For this review, take the finished solid that the model builds, in its own axes (mm). A direction names the side the tool comes from. Coordinates: 2 decimals unless noted, no trailing zeros. Order: outer loops, then holes, each group sorted by start corner. A loop starts at its lowest first (then second) coordinate and runs counter-clockwise, first axis right, second up. Notation, with made-up numbers: (34.25, -29) -> (88.25, -29) arc R27 cw to (88.25, -12) -> close; hole circle Ø5 at (-6, 84.25). An arc over 180 degrees is marked (long way). Return JSON: item names as keys, results as strings. Group by question number.
Item 1: Take a section at A-A (y = -5). Write out the cut boundary in (x, z).
Item 2: Take a section at D-D (z = 16.5). Write out the cut boundary in (x, y), then the cut area to 3 significant figures.
Item 3: Take a section at B-B (z = 3.25). Count the separate pieces of the cut face and the enclosed holes in it, then the cut area to 3 significant figures.
Item 4: For line 1 along Y through (x, z) = (-25, 11.75); line 2 along Y through (x, z) = (-15.5, 3.5); line 3 along X through (y, z) = (-17, 10.25), list the stretches that pass through material, from the lowest coordinate up.
Item 5: Take a section at C-C (x = -52). Write out the cut boundary in (y, z), then the cut area to 3 significant figures.
Item 6: Machinability: for faces 1 (the flat face through (9, 10, 8)), 2 (the flat face through (-39, 13, 4)), 3 (the flat face through (7.15, -26, 10)), which of the approach directions +Z, -Z, +X, -X, +Y, -Y give a long, thin tool a straight path to every point of the face, cutting with its end or side? Answer none if there is none.
Item 7: Draft analysis for pull direction Y (two halves, no side actions). For faces 4 (the flat face through (21, 0, 4)), 5 (the cylindrical face through (-50.522, 9.466, 7.395)), 6 (the flat face through (-34, -21, 4)), state which applies: +Y half, -Y half, draft (parallel to the pull), parting line (faces both ways), or undercut.
Item 8: Insertion check: pin 1 (6.5 mm diameter, centred on x = 15.5, z = 4, fed in from -Y); pin 2 (12.5 mm diameter, centred on x = -6, y = -10, fed in from +Z); pin 3 (1.5 mm diameter, centred on y = -11, z = 12.5, fed in from +X). Each pin has a flat end and moves straight along its axis. Give the tip position at first contact, or say it passes through.
```python
from build123d import *

# Parameters (mm, degrees)
F0_R     = 1.5
F0_R_2   = 13
F0_W     = 35
F0_H     = 34
F0_R_3   = 1.55
F1_DEPTH = 8
F2_W     = 18.5
F2_H     = 8
F2_R     = 4.25
F3_DEPTH = 10
F5_DEPTH = 34
F6_DEPTH = 42.001
F7_DEPTH = 28.751


with BuildPart() as f1:
    # F0 (on Top) → F1 (new body)
    with BuildSketch(Plane.XY):
        Polygon((21, 21), (-21, 21), (-21, 13), (-21, -21), (0, -21), (21, -21), (21, -16), align=None)
        with Locations((-15.5, -15.5)):
            Circle(F0_R, mode=Mode.SUBTRACT)
        with Locations((15.5, -15.5)):
            Circle(F0_R, mode=Mode.SUBTRACT)
        Circle(F0_R_2, mode=Mode.SUBTRACT)
        with Locations((-15.5, 15.5)):
            Circle(F0_R, mode=Mode.SUBTRACT)
        with Locations((15.5, 15.5)):
            Circle(F0_R, mode=Mode.SUBTRACT)
        with Locations((-38.5, -4)):
            Rectangle(F0_W, F0_H)
        with Locations((-52, -17)):
            Circle(F0_R_3, mode=Mode.SUBTRACT)
        with Locations((-25, -17)):
            Circle(F0_R_3, mode=Mode.SUBTRACT)
        with Locations((-52, 9)):
            Circle(F0_R_3, mode=Mode.SUBTRACT)
        with Locations((-25, 9)):
            Circle(F0_R_3, mode=Mode.SUBTRACT)
    extrude(amount=F1_DEPTH)

    # F2 (on face) → F3 (join)
    with BuildSketch(Plane.XZ.offset(21)):
        with Locations((-2.1, 4)):
            Rectangle(F2_W, F2_H)
        with BuildLine():
            Line((-11.35, 19.5), (-11.35, 8))
            Line((-11.35, 8), (7.15, 8))
            Line((7.15, 8), (7.15, 19.5))
            ThreePointArc((7.15, 19.5), (-2.1, 28.75), (-11.35, 19.5))
        make_face()
        with Locations((-2.1, 19.5)):
            Circle(F2_R, mode=Mode.SUBTRACT)
    extrude(amount=F3_DEPTH)

    # F4 (on face) → F5 (join, through all)
    with BuildSketch(Plane.XZ.offset(21)):
        with BuildLine():
            Line((-56, 15), (-56, 8))
            Line((-56, 8), (-46.4874895659, 8))
            ThreePointArc((-46.4874895659, 8), (-48.5343921686, 11.2373060217), (-49.25, 15))
            Line((-49.25, 15), (-56, 15))
        make_face()
        with BuildLine():
            ThreePointArc((-28.75, 15), (-29.4656078314, 11.2373060217), (-31.5125104341, 8))
            Line((-31.5125104341, 8), (-22, 8))
            Line((-22, 8), (-22, 15))
            Line((-22, 15), (-28.75, 15))
        make_face()
    extrude(amount=-F5_DEPTH)

    # F4 (on face) → F6 (cut, through all)
    with BuildSketch(Plane.XZ.offset(21)):
        with BuildLine():
            Line((-31.5125104341, 8), (-46.4874895659, 8))
            ThreePointArc((-46.4874895659, 8), (-39, 4.75), (-31.5125104341, 8))
        make_face()
    extrude(amount=-F6_DEPTH, mode=Mode.SUBTRACT)

    # F0 (on Top) → F7 (cut, through all)
    with BuildSketch(Plane.XY):
        with Locations((-52, -17)):
            Circle(F0_R_3)
        with Locations((-25, -17)):
            Circle(F0_R_3)
        with Locations((-25, 9)):
            Circle(F0_R_3)
        with Locations((-52, 9)):
            Circle(F0_R_3)
    extrude(amount=F7_DEPTH, mode=Mode.SUBTRACT)


solid = f1.part
```
Findings below:
{
 "1": {"outline": "(-56, 0) -> (-12, 0) -> (-12, 8) -> (-22, 8) -> (-22, 15) -> (-28.75, 15) arc R10.25 cw to (-49.25, 15) -> (-56, 15) -> close; (12, 0) -> (21, 0) -> (21, 8) -> (12, 8) -> close"},
 "2": {"outline": "(-11.35, -31) -> (-5.11, -31) -> (-5.11, -21) -> (-11.35, -21) -> close; (0.91, -31) -> (7.15, -31) -> (7.15, -21) -> (0.91, -21) -> close", "area": "125 mm2"},
 "3": {"separate pieces": "1", "enclosed holes": "9", "area": "2,550 mm2"},
 "4": {"line 1": "y = -21 to -18.55, -15.45 to 7.45, 10.55 to 13", "line 2": "y = -21 to -17, -14 to 14, 17 to 21", "line 3": "x = -56 to -53.55, -50.45 to -48.08, -29.92 to -26.55, -23.45 to -22"},
 "5": {"outline": "(-21, 0) -> (-18.55, 0) -> (-18.55, 15) -> (-21, 15) -> close; (-15.45, 0) -> (7.45, 0) -> (7.45, 15) -> (-15.45, 15) -> close; (10.55, 0) -> (13, 0) -> (13, 15) -> (10.55, 15) -> close", "area": "417 mm2"},
 "6": {"face 1": "+Z, +X, +Y", "face 2": "+Z, -Z, -X, +Y", "face 3": "+Z, -Z, +X, -Y"},
 "7": {"face 4": "draft", "face 5": "undercut", "face 6": "-Y half"},
 "8": {"pin 1": "stops at y = -21", "pin 2": "stops at z = 8", "pin 3": "stops at x = -22"}
}
